Read the model definition and answer for the solid it produces. Units are mm, in the model's axes. Round coordinates to 2 decimals unless told otherwise and drop trailing zeros. Order: outer loops, then holes, each group sorted by start corner. A loop starts at its lowest first (then second) coordinate and runs counter-clockwise, first axis right, second up. Notation, with made-up numbers: (75.5, 62.25) -> (112.5, 62.25) arc R22 cw to (112.5, 89.25) -> close; hole circle Ø2 at (5.25, 66.5). An arc over 180 degrees is marked (long way). Answer as a JSON object with one key per item and string values. Group by question number.
Item 1: Given P1, Ø1.5, axis at y = 58, z = 1.5, coming from the -X side; P2, Ø1.5, axis at x = 103, z = 2, coming from the -Y side; P3, Ø1.5, axis at y = -56.5, z = 2.5, coming from the +X side; P4, Ø12, axis at x = 80.5, y = 43, coming from the +Z side, each flat-ended and moving along its own axis, determine where each tip first touches the part or whether it passes through.
Item 2: Section A-A, the plane x = -83.5 is taken. Write down the section's boundary in (y, z), plus the area to 3 significant figures.
Item 3: Section B-B, the plane y = -21 is taken. Write down the section's boundary in (x, z), plus the area to 3 significant figures.
Item 4: Consider probe 1 along Y at (x, z) = (88, 3.8); probe 2 along X at (y, z) = (6, 4.4); probe 3 along Y at (x, z) = (-38.5, 4.3). Determine where each line is inside the solid, lowest interval first. Write a range as from..to.
Autodesk Inventor part; units mm, degrees
ref_plane "YZ Plane" through (0, 0, 0) normal (1, 0, 0) x (0, 1, 0)
ref_plane "XZ Plane" through (0, 0, 0) normal (0, 1, 0) x (-1, 0, 0)
ref_plane "XY Plane" through (0, 0, 0) normal (0, 0, 1) x (1, 0, 0)
sketch "Sketch1" plane through (0, 0, 0) normal (0, 0, 1) x (1, 0, 0)
  line L0 (-105, -65) -> (105, -65)
  line L1 (105, -65) -> (105, 65)
  line L2 (105, 65) -> (-105, 65)
  line L3 (-105, 65) -> (-105, -65)
  line L4 (-105, -65) -> (105, 65) construction
  line L5 (105, -65) -> (-105, 65) construction
  line L6 (-88.5, -51) -> (88.5, -51)
  line L7 (88.5, -51) -> (88.5, 51)
  line L8 (88.5, 51) -> (-88.5, 51)
  line L9 (-88.5, 51) -> (-88.5, -51)
  line L10 (-88.5, -51) -> (88.5, 51) construction
  line L11 (88.5, -51) -> (-88.5, 51) construction
  point P0 (0, 0)
  point P1 (-105, 0)
  dimension "d0" = 177
  dimension "d1" = 102
  dimension "d2" = 130
  dimension "d3" = 210
extrude "Extrusion1" add sketch "Sketch1" along normal blind 5 contours L3 L2 L1 L0 | L9 L8 L7 L6
sketch "Sketch2" plane through (0, 0, 5) normal (0, 0, 1) x (1, 0, 0)
  line L0 (-90, -50) -> (-80, -50) construction
  line L1 (-80, -50) -> (-80, 50)
  line L2 (-80, 50) -> (-90, 50) construction
  line L3 (-90, 50) -> (-90, -50)
  line L4 (-90, -50) -> (-80, 50) construction
  line L5 (-80, -50) -> (-90, 50) construction
  line L6 (-105, 65) -> (-105, -65) construction
  line L7 (-88.5, -51) -> (-88.5, 51) construction
  arc A0 (-80, 50) -> (-90, 50) centre (-85, 50) ccw
  arc A1 (-90, -50) -> (-80, -50) centre (-85, -50) ccw
  point P0 (0, 0)
  point P1 (-85, 0)
  dimension "d6" = 10
  dimension "d7" = 100
  dimension "d10" = 20
extrude "Extrusion2" [suppressed]
mirror "Mirror1" [suppressed]
sketch "Sketch3" plane through (0, 0, 0) normal (0, 0, -1) x (-1, 0, 0)
  line L0 (105, -65) -> (99.9, -65)
  line L1 (99.9, -65) -> (99.9, -38.95)
  line L2 (99.9, -38.95) -> (105, -38.95)
  line L3 (105, -38.95) -> (105, -65)
  line L4 (105, -13.05) -> (99.9, -13.05)
  line L5 (99.9, -13.05) -> (99.9, 13.05)
  line L6 (99.9, 13.05) -> (105, 13.05)
  line L7 (105, 13.05) -> (105, -13.05)
  line L8 (105, 65) -> (99.9, 65)
  line L9 (99.9, 65) -> (99.9, 38.95)
  line L10 (99.9, 38.95) -> (105, 38.95)
  line L11 (105, 38.95) -> (105, 65)
  line L12 (-105, -65) -> (-105, 65)
  line L13 (-105, 65) -> (-99.9, 65)
  line L14 (-99.9, 65) -> (-99.9, 38.95)
  line L15 (-99.9, 38.95) -> (-105, 38.95)
  line L16 (-105, 38.95) -> (-105, 65)
  line L17 (-105, 13.05) -> (-99.9, 13.05)
  line L18 (-99.9, 13.05) -> (-99.9, -13.05)
  line L19 (-99.9, -13.05) -> (-105, -13.05)
  line L20 (-105, -13.05) -> (-105, 13.05)
  line L21 (-105, -65) -> (-99.9, -65)
  line L22 (-99.9, -65) -> (-99.9, -38.95)
  line L23 (-99.9, -38.95) -> (-105, -38.95)
  line L24 (-105, -38.95) -> (-105, -65)
  line L25 (105, -65) -> (-105, -65)
  line L26 (-105, 65) -> (105, 65)
  point P0 (0, 0)
  point P1 (-105, 0)
  point P2 (-105, -13.05)
  dimension "d13" = 130
  dimension "d14" = 26.05
  dimension "d15" = 26.1
  dimension "d16" = 5.1
extrude "Extrusion3" cut sketch "Sketch3" against normal blind 10
sketch "Sketch4" plane through (-99.9, -65, 0) normal (0, -1, 0) x (1, 0, 0)
  line L0 (0, 5) -> (0, 0)
  line L1 (0, 0) -> (199.8, 0)
  line L2 (199.8, 0) -> (199.8, 5)
  line L3 (0, 5) -> (199.8, 5)
  point P0 (99.9, 0)
extrude "Extrusion4" add sketch "Sketch4" along normal blind 2
sketch "Sketch5" plane through (0, 0, 0) normal (0, 0, -1) x (-1, 0, 0)
  line L0 (99.9, 38.95) -> (99.9, 65)
  line L1 (-99.9, 65) -> (99.9, 65)
  line L2 (-99.9, 65) -> (-99.9, 38.95)
  line L3 (-99.9, 38.95) -> (-105, 38.95)
  line L4 (-105, 13.05) -> (-105, 38.95)
  line L5 (-105, 13.05) -> (-99.9, 13.05)
  line L6 (-99.9, 13.05) -> (-99.9, -13.05)
  line L7 (-99.9, -13.05) -> (-105, -13.05)
  line L8 (-105, -38.95) -> (-105, -13.05)
  line L9 (-105, -38.95) -> (-99.9, -38.95)
  line L10 (-99.9, -38.95) -> (-99.9, -67)
  line L11 (99.9, -67) -> (99.9, -38.95)
  line L12 (99.9, -38.95) -> (105, -38.95)
  line L13 (105, -13.05) -> (105, -38.95)
  line L14 (105, -13.05) -> (99.9, -13.05)
  line L15 (99.9, -13.05) -> (99.9, 13.05)
  line L16 (99.9, 13.05) -> (105, 13.05)
  line L17 (105, 38.95) -> (105, 13.05)
  line L18 (105, 38.95) -> (99.9, 38.95)
  line L19 (8.65, -67) -> (26.25, -67)
  line L20 (26.25, -67) -> (26.25, -61.4)
  line L21 (26.25, -61.4) -> (8.65, -61.4)
  line L22 (8.65, -61.4) -> (8.65, -67)
  line L23 (43.65, -61.4) -> (43.65, -67)
  line L24 (43.65, -67) -> (61.25, -67)
  line L25 (61.25, -61.4) -> (43.65, -61.4)
  line L26 (61.25, -67) -> (61.25, -61.4)
  line L27 (78.65, -61.4) -> (78.65, -67)
  line L28 (78.65, -67) -> (96.25, -67)
  line L29 (96.25, -61.4) -> (78.65, -61.4)
  line L30 (96.25, -67) -> (96.25, -61.4)
  line L31 (0, 0) -> (0, -124.7) construction
  line L32 (150.9327, -2.5) -> (-150.9327, -2.5) construction
  line L33 (-8.65, -67) -> (-26.25, -67)
  line L34 (-26.25, -67) -> (-26.25, -61.4)
  line L35 (-26.25, -61.4) -> (-8.65, -61.4)
  line L36 (-8.65, -61.4) -> (-8.65, -67)
  line L37 (-43.65, -61.4) -> (-43.65, -67)
  line L38 (-43.65, -67) -> (-61.25, -67)
  line L39 (-61.25, -61.4) -> (-43.65, -61.4)
  line L40 (-61.25, -67) -> (-61.25, -61.4)
  line L41 (-78.65, -61.4) -> (-78.65, -67)
  line L42 (-78.65, -67) -> (-96.25, -67)
  line L43 (-96.25, -61.4) -> (-78.65, -61.4)
  line L44 (-96.25, -67) -> (-96.25, -61.4)
  line L45 (99.9, -67) -> (-99.9, -67)
  line L46 (99.9, -67) -> (-99.9, -67)
  point P0 (17.45, -61.4)
  point P1 (52.45, -61.4)
  point P2 (87.45, -61.4)
  point P3 (0, -2.5)
  point P4 (-17.45, -61.4)
  point P5 (-52.45, -61.4)
  point P6 (-87.45, -61.4)
  dimension "d21" = 210
  dimension "d22" = 17.45
  dimension "d23" = 17.6
  dimension "d24" = 5.6
  dimension "d27" = 35
extrude "Extrusion5" cut sketch "Sketch5" against normal through all contours L28 L27 L29 L30 | L24 L23 L25 L26 | L44 L43 L41 L42 | L19 L22 L21 L20 | L40 L39 L37 L38 | L33 L34 L35 L36
sketch "Sketch7" plane through (0, 0, 0) normal (0, 0, -1) x (-1, 0, 0)
  line L0 (99.9, 53) -> (-99.9, 53) construction
  line L1 (8.65, 53) -> (26.25, 53)
  line L2 (26.25, 53) -> (26.25, 65)
  line L3 (26.25, 65) -> (8.65, 65)
  line L4 (8.65, 65) -> (8.65, 53)
  line L5 (43.65, 65) -> (43.65, 53)
  line L6 (43.65, 53) -> (61.25, 53)
  line L7 (61.25, 65) -> (43.65, 65)
  line L8 (61.25, 53) -> (61.25, 65)
  line L9 (78.65, 65) -> (78.65, 53)
  line L10 (78.65, 53) -> (96.25, 53)
  line L11 (96.25, 65) -> (78.65, 65)
  line L12 (96.25, 53) -> (96.25, 65)
  line L13 (99.9, 38.95) -> (99.9, 65)
  line L14 (-99.9, 65) -> (-99.9, 38.95)
  line L15 (-99.9, 65) -> (99.9, 65)
  line L16 (0, 0) -> (0, 28.7468) construction
  line L17 (-43.65, 65) -> (-43.65, 53)
  line L18 (-43.65, 53) -> (-61.25, 53)
  line L19 (-61.25, 65) -> (-43.65, 65)
  line L20 (-61.25, 53) -> (-61.25, 65)
  line L21 (-78.65, 65) -> (-78.65, 53)
  line L22 (-96.25, 65) -> (-78.65, 65)
  line L23 (-78.65, 53) -> (-96.25, 53)
  line L24 (-96.25, 53) -> (-96.25, 65)
  line L25 (-8.65, 53) -> (-26.25, 53)
  line L26 (-26.25, 53) -> (-26.25, 65)
  line L27 (-8.65, 65) -> (-8.65, 53)
  line L28 (-26.25, 65) -> (-8.65, 65)
  point P0 (0, 53)
  point P1 (17.45, 65)
  point P2 (52.45, 65)
  point P3 (87.45, 65)
  point P4 (-52.45, 65)
  point P5 (-87.45, 65)
  point P6 (-17.45, 65)
  dimension "d41" = 17.45
  dimension "d42" = 17.6
  dimension "d44" = 35
  dimension "d47" = 12
extrude "Extrusion7" cut sketch "Sketch7" against normal blind 10
sketch "Sketch8" plane through (0, 0, 0) normal (0, 0, -1) x (-1, 0, 0)
  line L0 (26.25, 65) -> (26.25, 53)
  line L1 (26.25, 53) -> (8.65, 53)
  line L2 (8.65, 53) -> (8.65, 65)
  line L3 (-8.65, 65) -> (8.65, 65)
  line L4 (-8.65, 65) -> (-8.65, 53)
  line L5 (-8.65, 53) -> (-26.25, 53)
  line L6 (-26.25, 53) -> (-26.25, 65)
  line L7 (-43.65, 65) -> (-26.25, 65)
  line L8 (-43.65, 65) -> (-43.65, 53)
  line L9 (-43.65, 53) -> (-61.25, 53)
  line L10 (-61.25, 53) -> (-61.25, 65)
  line L11 (-78.65, 65) -> (-61.25, 65)
  line L12 (-78.65, 65) -> (-78.65, 53)
  line L13 (-78.65, 53) -> (-96.25, 53)
  line L14 (-96.25, 53) -> (-96.25, 65)
  line L15 (-99.9, 65) -> (-96.25, 65)
  line L16 (-99.9, 65) -> (-99.9, 38.95)
  line L17 (-99.9, 38.95) -> (-105, 38.95)
  line L18 (-105, 13.05) -> (-105, 38.95)
  line L19 (-105, 13.05) -> (-99.9, 13.05)
  line L20 (-99.9, 13.05) -> (-99.9, -13.05)
  line L21 (-99.9, -13.05) -> (-105, -13.05)
  line L22 (-105, -38.95) -> (-105, -13.05)
  line L23 (-105, -38.95) -> (-99.9, -38.95)
  line L24 (-99.9, -38.95) -> (-99.9, -67)
  line L25 (-96.25, -67) -> (-99.9, -67)
  line L26 (-96.25, -67) -> (-96.25, -61.4)
  line L27 (-96.25, -61.4) -> (-78.65, -61.4)
  line L28 (-78.65, -61.4) -> (-78.65, -67)
  line L29 (-61.25, -67) -> (-78.65, -67)
  line L30 (-61.25, -67) -> (-61.25, -61.4)
  line L31 (-61.25, -61.4) -> (-43.65, -61.4)
  line L32 (-43.65, -61.4) -> (-43.65, -67)
  line L33 (-26.25, -67) -> (-43.65, -67)
  line L34 (-26.25, -67) -> (-26.25, -61.4)
  line L35 (-26.25, -61.4) -> (-8.65, -61.4)
  line L36 (-8.65, -61.4) -> (-8.65, -67)
  line L37 (8.65, -67) -> (-8.65, -67)
  line L38 (8.65, -67) -> (8.65, -61.4)
  line L39 (8.65, -61.4) -> (26.25, -61.4)
  line L40 (26.25, -61.4) -> (26.25, -67)
  line L41 (43.65, -67) -> (26.25, -67)
  line L42 (43.65, -67) -> (43.65, -61.4)
  line L43 (43.65, -61.4) -> (61.25, -61.4)
  line L44 (61.25, -61.4) -> (61.25, -67)
  line L45 (78.65, -67) -> (61.25, -67)
  line L46 (78.65, -67) -> (78.65, -61.4)
  line L47 (78.65, -61.4) -> (96.25, -61.4)
  line L48 (96.25, -61.4) -> (96.25, -67)
  line L49 (99.9, -67) -> (96.25, -67)
  line L50 (99.9, -67) -> (99.9, -38.95)
  line L51 (99.9, -38.95) -> (105, -38.95)
  line L52 (105, -13.05) -> (105, -38.95)
  line L53 (105, -13.05) -> (99.9, -13.05)
  line L54 (99.9, -13.05) -> (99.9, 13.05)
  line L55 (99.9, 13.05) -> (105, 13.05)
  line L56 (105, 38.95) -> (105, 13.05)
  line L57 (105, 38.95) -> (99.9, 38.95)
  line L58 (99.9, 38.95) -> (99.9, 65)
  line L59 (96.25, 65) -> (99.9, 65)
  line L60 (96.25, 65) -> (96.25, 53)
  line L61 (96.25, 53) -> (78.65, 53)
  line L62 (78.65, 53) -> (78.65, 65)
  line L63 (61.25, 65) -> (78.65, 65)
  line L64 (61.25, 65) -> (61.25, 53)
  line L65 (61.25, 53) -> (43.65, 53)
  line L66 (43.65, 53) -> (43.65, 65)
  line L67 (26.25, 65) -> (43.65, 65)
  line L68 (99.9, 60) -> (-99.9, 60)
  point P0 (0, 0)
  point P1 (-99.9, -62)
  point P2 (99.9, -62)
  point P3 (-98.075, -67)
  point P4 (-98.075, 65)
  point P5 (-8.65, 60)
  point P6 (8.65, 60)
  point P7 (-43.65, 60)
  point P8 (-26.25, 60)
  point P9 (-78.65, 60)
  point P10 (-61.25, 60)
  point P11 (-96.25, 60)
  point P12 (96.25, 60)
  point P13 (61.25, 60)
  point P14 (78.65, 60)
  point P15 (26.25, 60)
  point P16 (43.65, 60)
  dimension "d53" = 5
extrude "Extrusion8" cut sketch "Sketch8" against normal through all contours L67 L66 L68 L0 | L68 L4 L3 L2 | L64 L63 L62 L68 | L68 L8 L7 L6 | L60 L59 L58 L68 | L68 L12 L11 L10 | L68 L16 L15 L14
sketch "Sketch9" plane through (0, 0, 0) normal (0, 0, -1) x (-1, 0, 0)
  line L0 (88.5, -55.2) -> (-88.5, -55.2)
  line L1 (-88.5, -55.2) -> (-88.5, 46.8)
  line L2 (-88.5, 46.8) -> (88.5, 46.8)
  line L3 (88.5, 46.8) -> (88.5, -55.2)
  line L4 (88.5, -55.2) -> (-88.5, 46.8) construction
  line L5 (-88.5, -55.2) -> (88.5, 46.8) construction
  line L6 (-8.65, 60) -> (8.65, 60)
  line L7 (8.65, -67) -> (-8.65, -67)
  line L8 (8.65, 53) -> (26.25, 53)
  line L9 (17.45, 53) -> (-17.45, -61.4)
  line L10 (-8.65, -61.4) -> (-26.25, -61.4)
  point P0 (0, 0)
  point P1 (0, -4.2)
  dimension "d54" = 177
  dimension "d55" = 102
extrude "Extrusion9" cut sketch "Sketch9" against normal blind 5
equation "\"d27\" = 0.166667 * d21"
equation "\"d44\" = 0.166667 * d46"
properties part number "Frontplate" material "MDF Medium Density Fiberboard"
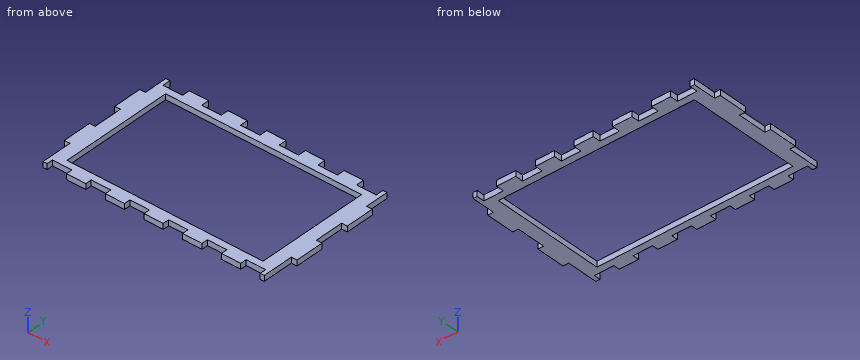
Values found:
{
 "1": {"P1": "x = -99.9", "P2": "y = -38.95", "P3": "x = 99.9", "P4": "z = 5"},
 "2": {"outline": "(-61.4, 0) -> (-55.2, 0) -> (-55.2, 5) -> (-61.4, 5) -> close; (46.8, 0) -> (53, 0) -> (53, 5) -> (46.8, 5) -> close", "area": "62.0 mm2"},
 "3": {"outline": "(-105, 0) -> (-88.5, 0) -> (-88.5, 5) -> (-105, 5) -> close; (88.5, 0) -> (105, 0) -> (105, 5) -> (88.5, 5) -> close", "area": "165 mm2"},
 "4": {"probe 1": "-61.4..-55.2, 46.8..53", "probe 2": "-99.9..-88.5, 88.5..99.9", "probe 3": "-67..-55.2, 46.8..60"}
}
